from build123d import *

# Parameters (mm, degrees)
EXTRUDE_1_DEPTH       = 1.5
SKETCH_2_R            = 6
CUT_EXTRUDE_1_DEPTH   = 0.1
SKETCH_11_R           = 2
SKETCH_11_W           = 12.230000073
SKETCH_11_H           = 11.974599949
EXTRUDE_5_DEPTH       = 1.539974634
SKETCH_13_R           = 2
SKETCH_13_W           = 4
SKETCH_13_H           = 10
TYPEC_2_DEPTH         = 4.7999746
LED_3_START           = -3.75
LED_3_DEPTH           = 2.25
LED_1_R               = 0.5
CUT_EXTRUDE_2_REACH   = 75.671
SKETCH_15_R           = 2
EXTRUDE_START         = -3
SKETCH_16_R           = 4
SKETCH_16_R_2         = 1
EXTRUDE_4_DEPTH       = 1.5
CUT_EXTRUDE_START     = -1.5
SKETCH_17_W           = 1
SKETCH_17_H           = 6
CUT_EXTRUDE_2_2_DEPTH = 0.5
SKETCH_18_W           = 40
SKETCH_18_H           = 3
EXTRUDE_2_DEPTH       = 2.5


with BuildPart() as part:
    # 草图1 → 凸台-拉伸1 (new body)
    with BuildSketch(Plane(origin=(0, 0, 0), x_dir=(1, 0, 0), z_dir=(0, 1, 0))):
        Polygon((-51.714401712, -9.454370264), (-55.816720774, -9.454370264), (-55.816720774, -21.428970213), (-51.714401712, -21.428970213), (-51.714401712, -47.841670238), (46.085598288, -47.841670238), (46.085598288, 16.958329762), (-51.714401712, 16.958329762), align=None)
    extrude(amount=EXTRUDE_1_DEPTH)

    # 草图2 → 切除-拉伸1 (cut)
    with BuildSketch(Plane.XZ):
        with Locations(Location((-43.814401712, -9.058329762, 0), (0, 0, 270))):
            Circle(SKETCH_2_R)
        with Locations(Location((-43.814401712, 39.941670238, 0), (0, 0, 270))):
            Circle(SKETCH_2_R)
        with Locations(Location((38.085598288, -9.058329762, 0), (0, 0, 270))):
            Circle(SKETCH_2_R)
        with Locations(Location((38.085598288, 39.941670238, 0), (0, 0, 270))):
            Circle(SKETCH_2_R)
    extrude(amount=-CUT_EXTRUDE_1_DEPTH, mode=Mode.SUBTRACT)

    # 草图11 → 充电板档板凸台-拉伸5 (add)
    with BuildSketch(Plane.XZ):
        with Locations((-28.914401712, 29.928970213)):
            Circle(SKETCH_11_R)
        with Locations((-28.914401712, 0.954370264)):
            Circle(SKETCH_11_R)
        with Locations((-49.701720738, 15.441670239)):
            Rectangle(SKETCH_11_W, SKETCH_11_H)
    extrude(amount=-EXTRUDE_5_DEPTH)

    # 草图13 → TypeC支撑凸台-拉伸2 (add)
    with BuildSketch(Plane.XZ):
        with Locations(Location((-28.914401712, 29.928970213, 0), (0, 0, 90))):
            Circle(SKETCH_13_R)
        with Locations(Location((-28.914401712, 0.954370264, 0), (0, 0, 90))):
            Circle(SKETCH_13_R)
        with Locations((-46.466720701, 15.441670238)):
            Rectangle(SKETCH_13_W, SKETCH_13_H)
    extrude(amount=-TYPEC_2_DEPTH)

    # 草图14 → LED限位凸台-拉伸3 (add)
    with BuildSketch(Plane.XZ.offset(LED_3_START)):
        Polygon((45.085598288, 12.441670238), (45.085598288, 18.441670238), (46.085598288, 18.441670238), (46.085598288, 21.441670238), (42.085598288, 21.441670238), (42.085598288, 9.441670238), (46.085598288, 9.441670238), (46.085598288, 12.441670238), align=None)
    extrude(amount=LED_3_DEPTH)

    # LED限位圆角1
    led_1_edges = [part.edges().sort_by_distance(p)[0] for p in [
        (45.585598288, 3.75, 18.441670238),
        (45.585598288, 3.75, 12.441670238),
        (45.085598288, 3.75, 15.441670238),
        (-48.466720701, 4.7999746, 15.441670238),
    ]]
    fillet(led_1_edges, radius=LED_1_R)

    # 草图15 → Cut-Extrude 2 (cut, up to next)
    with BuildSketch(Plane.XZ, mode=Mode.PRIVATE) as cut_extrude_2_sk1:
        with Locations(Location((-43.814401712, -9.058329762, 0), (0, 0, 270))):
            Circle(SKETCH_15_R)
    cut_extrude_2_tool1 = extrude(cut_extrude_2_sk1.sketch, amount=-CUT_EXTRUDE_2_REACH, mode=Mode.PRIVATE) & part.part
    # 草图15 → Cut-Extrude 2 (cut, up to next)
    with BuildSketch(Plane.XZ, mode=Mode.PRIVATE) as cut_extrude_2_sk2:
        with Locations(Location((-43.814401712, 39.941670238, 0), (0, 0, 270))):
            Circle(SKETCH_15_R)
    cut_extrude_2_tool2 = extrude(cut_extrude_2_sk2.sketch, amount=-CUT_EXTRUDE_2_REACH, mode=Mode.PRIVATE) & part.part
    # 草图15 → Cut-Extrude 2 (cut, up to next)
    with BuildSketch(Plane.XZ, mode=Mode.PRIVATE) as cut_extrude_2_sk3:
        with Locations(Location((38.085598288, 39.941670238, 0), (0, 0, 270))):
            Circle(SKETCH_15_R)
    cut_extrude_2_tool3 = extrude(cut_extrude_2_sk3.sketch, amount=-CUT_EXTRUDE_2_REACH, mode=Mode.PRIVATE) & part.part
    # 草图15 → Cut-Extrude 2 (cut, up to next)
    with BuildSketch(Plane.XZ, mode=Mode.PRIVATE) as cut_extrude_2_sk4:
        with Locations(Location((38.085598288, -9.058329762, 0), (0, 0, 270))):
            Circle(SKETCH_15_R)
    cut_extrude_2_tool4 = extrude(cut_extrude_2_sk4.sketch, amount=-CUT_EXTRUDE_2_REACH, mode=Mode.PRIVATE) & part.part
    add(cut_extrude_2_tool1.solids().sort_by_distance((-43.814402, 0, -9.05833))[0], mode=Mode.SUBTRACT)
    add(cut_extrude_2_tool2.solids().sort_by_distance((-43.814402, 0, 39.94167))[0], mode=Mode.SUBTRACT)
    add(cut_extrude_2_tool3.solids().sort_by_distance((38.085598, 0, 39.94167))[0], mode=Mode.SUBTRACT)
    add(cut_extrude_2_tool4.solids().sort_by_distance((38.085598, 0, -9.05833))[0], mode=Mode.SUBTRACT)

    # 草图16 → 螺丝孔凸台-拉伸4 (add)
    # profile 1 of 4: a face of its own
    with BuildSketch(Plane.XZ.offset(EXTRUDE_START)):
        with Locations((38.085598288, 39.941670238)):
            Circle(SKETCH_16_R)
        with Locations((38.085598288, 39.941670238)):
            Circle(SKETCH_16_R_2, mode=Mode.SUBTRACT)
    # profile 2 of 4: a face of its own
    with BuildSketch(Plane.XZ.offset(EXTRUDE_START)):
        with Locations((38.085598288, -9.058329762)):
            Circle(SKETCH_16_R)
        with Locations((38.085598288, -9.058329762)):
            Circle(SKETCH_16_R_2, mode=Mode.SUBTRACT)
    # profile 3 of 4: a face of its own
    with BuildSketch(Plane.XZ.offset(EXTRUDE_START)):
        with Locations((-43.814401712, -9.058329762)):
            Circle(SKETCH_16_R)
        with Locations((-43.814401712, -9.058329762)):
            Circle(SKETCH_16_R_2, mode=Mode.SUBTRACT)
    # profile 4 of 4: a face of its own
    with BuildSketch(Plane.XZ.offset(EXTRUDE_START)):
        with Locations((-43.814401712, 39.941670238)):
            Circle(SKETCH_16_R)
        with Locations((-43.814401712, 39.941670238)):
            Circle(SKETCH_16_R_2, mode=Mode.SUBTRACT)
    extrude(amount=EXTRUDE_4_DEPTH)

    # 草图17 → Cut-Extrude 2 2 (cut)
    with BuildSketch(Plane.XZ.offset(CUT_EXTRUDE_START)):
        with Locations((45.585598288, 15.441670238)):
            Rectangle(SKETCH_17_W, SKETCH_17_H)
    extrude(amount=CUT_EXTRUDE_2_2_DEPTH, mode=Mode.SUBTRACT)

    # 草图18 → 凸台-拉伸2 (add)
    with BuildSketch(Plane(origin=(0, 1.5, 0), x_dir=(1, 0, 0), z_dir=(0, 1, 0))):
        with Locations((-5.814401712, 3.058329762)):
            Rectangle(SKETCH_18_W, SKETCH_18_H)
        with Locations((-5.814401712, -33.941670238)):
            Rectangle(SKETCH_18_W, SKETCH_18_H)
    extrude(amount=EXTRUDE_2_DEPTH)


solid = part.part
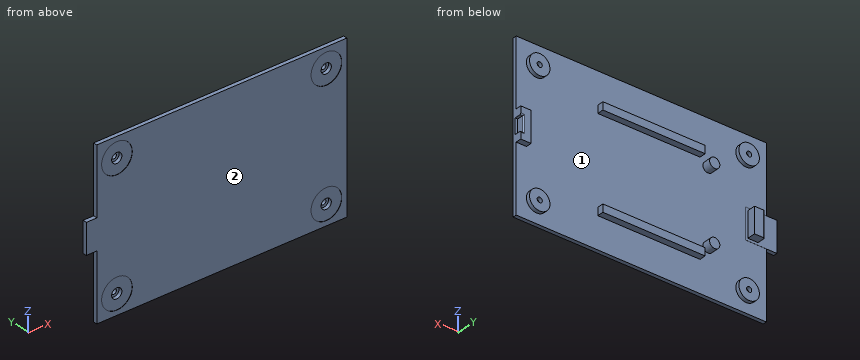
Geometry: final body of the model. Coordinates: model frame, mm. Face numbers are marked on the shaded views. Coordinates: 2 decimals unless noted, no trailing zeros. Order: outer loops, then holes, each group sorted by start corner. A loop starts at its lowest first (then second) coordinate and runs counter-clockwise, first axis right, second up.
1) Draft query along Z for the marked faces 1 and 2. Return one class per face: released by +Z, released by -Z, zero draft, split by the parting line, or undercut.
Result sheet:
face 1: undercut
face 2: zero draft
2) Section B-B (z = 22.5). Return loops of the section in (x, y), then the cut area to 3 significant figures.
Result sheet:
outline: (-51.71, 0) - (46.09, 0) - (46.09, 1.5) - (-51.71, 1.5) - close
area: 147 mm2
3) Section C-C (x = -34.5). Return loops of the section in (y, z).
Result sheet:
outline: (0, -16.96) - (1.5, -16.96) - (1.5, 47.84) - (0, 47.84) - close
4) Ray query, probe 1 along X at (y, z) = (1.9, 17.5); probe 2 along Z at (x, y) = (-18.5, 2.4); probe 3 along Y at (x, z) = (-39, 33). Return the intervals inside material, ascending.
Result sheet:
probe 1: x = -48.47 to -44.47, 42.09 to 45.09
probe 2: z = -4.56 to -1.56, 32.44 to 35.44
probe 3: y = 0 to 1.5
5) Section A-A (x = 6). Return loops of the section in (y, z), then the cut area to 3 significant figures.
Result sheet:
outline: (0, -16.96) - (1.5, -16.96) - (1.5, -4.56) - (4, -4.56) - (4, -1.56) - (1.5, -1.56) - (1.5, 32.44) - (4, 32.44) - (4, 35.44) - (1.5, 35.44) - (1.5, 47.84) - (0, 47.84) - close
area: 112 mm2
6) First-contact query: P1, Ø6, axis at x = 36.5, z = -9.5, coming from the -Y side; P2, Ø0.8, axis at y = 0.5, z = 2.5, coming from the -X side; P3, Ø2, axis at y = 4, z = 19, coming from the -X side. Flat tips, straight axial feed; report the tip coordinate or a pass-through.
Result sheet:
P1: stops at y = 0.1
P2: stops at x = -51.71
P3: stops at x = -48.47
